```python
from build123d import *

# Parameters (mm, degrees)
Y_KSEKLIK_EKSTR_ZYON5_DEPTH = 4
Y_KSEKLIK_EKSTR_ZYON6_DEPTH = 40
RADYUS2_R                   = 1
KES_EKSTR_ZYON1_DEPTH       = 4
KES_EKSTR_ZYON2_DEPTH       = 35


with BuildPart() as part:
    # Çizim1 → Yükseklik-Ekstrüzyon5 (new body)
    with BuildSketch(Plane.XY):
        with BuildLine():
            Line((20, 0), (95, 0))
            ThreePointArc((95, 0), (100.857864376, -14.142135624), (115, -20))
            Line((115, -20), (115, -95))
            ThreePointArc((115, -95), (111.464466094, -96.464466094), (110, -100))
            Line((110, -100), (110, -170))
            Line((110, -170), (5, -170))
            Line((5, -170), (5, -100))
            ThreePointArc((5, -100), (3.535533906, -96.464466094), (0, -95))
            Line((0, -95), (0, -20))
            ThreePointArc((0, -20), (14.142135624, -14.142135624), (20, 0))
        make_face()
    extrude(amount=Y_KSEKLIK_EKSTR_ZYON5_DEPTH)

    # Çizim6 → Yükseklik-Ekstrüzyon6 (add)
    with BuildSketch(Plane.XY.offset(4)):
        Polygon((33.5, -4), (81.5, -4), (109.784271247, -32.284271247), (109.784271247, -87.284271247), (102.713203436, -94.355339059), (102.713203436, -154.355339059), (93.52081528, -163.547727215), (21.47918472, -163.547727215), (12.286796564, -154.355339059), (12.286796564, -94.355339059), (5.215728753, -87.284271247), (5.215728753, -32.284271247), align=None)
    extrude(amount=Y_KSEKLIK_EKSTR_ZYON6_DEPTH)

    # Radyus2
    radyus2_edges = [part.edges().sort_by_distance(p)[0] for p in [
        (20, 0, 2),
        (95, 0, 2),
        (115, -20, 2),
        (115, -95, 2),
        (110, -170, 2),
        (5, -170, 2),
        (0, -95, 2),
        (0, -20, 2),
        (95.642135624, -18.142135624, 4),
        (109.784271247, -32.284271247, 24),
        (57.5, -4, 4),
        (81.5, -4, 24),
        (19.357864376, -18.142135624, 4),
        (33.5, -4, 24),
        (5.215728753, -59.784271247, 4),
        (5.215728753, -32.284271247, 24),
        (8.751262658, -90.819805153, 4),
        (5.215728753, -87.284271247, 24),
        (12.286796564, -124.355339059, 4),
        (12.286796564, -94.355339059, 24),
        (16.882990642, -158.951533137, 4),
        (12.286796564, -154.355339059, 24),
        (57.5, -163.547727215, 4),
        (21.47918472, -163.547727215, 24),
        (98.117009358, -158.951533137, 4),
        (93.52081528, -163.547727215, 24),
        (102.713203436, -124.355339059, 4),
        (102.713203436, -154.355339059, 24),
        (106.248737342, -90.819805153, 4),
        (102.713203436, -94.355339059, 24),
        (109.784271247, -59.784271247, 4),
        (109.784271247, -87.284271247, 24),
        (95.642135624, -18.142135624, 44),
        (57.5, -4, 44),
        (19.357864376, -18.142135624, 44),
        (5.215728753, -59.784271247, 44),
        (8.751262658, -90.819805153, 44),
        (12.286796564, -124.355339059, 44),
        (16.882990642, -158.951533137, 44),
        (57.5, -163.547727215, 44),
        (98.117009358, -158.951533137, 44),
        (102.713203436, -124.355339059, 44),
        (106.248737342, -90.819805153, 44),
        (109.784271247, -59.784271247, 44),
    ]]
    fillet(radyus2_edges, radius=RADYUS2_R)

    # Çizim8 → Kes-Ekstrüzyon1 (cut)
    with BuildSketch(Plane(origin=(0, 0, 0), x_dir=(-1, 0, 0), z_dir=(0, 0, -1))):
        Polygon((-81.5, -5), (-33.5, -5), (-5.215728753, -33.284271247), (-5.215728753, -88.284271247), (-12.286796564, -95.355339059), (-12.286796564, -153.355339059), (-21.47918472, -162.547727215), (-93.52081528, -162.547727215), (-102.713203436, -153.355339059), (-102.713203436, -95.355339059), (-109.784271247, -88.284271247), (-109.784271247, -33.284271247), align=None)
    extrude(amount=-KES_EKSTR_ZYON1_DEPTH, mode=Mode.SUBTRACT)

    # Çizim9 → Kes-Ekstrüzyon2 (cut)
    with BuildSketch(Plane(origin=(0, 0, 4), x_dir=(-1, 0, 0), z_dir=(0, 0, -1))):
        Polygon((-80.5, -7), (-34.5, -7), (-6.922835534, -34.577164466), (-6.922835534, -86.577164466), (-14.701010127, -94.355339059), (-14.701010127, -150.355339059), (-22.47918472, -158.133513652), (-92.52081528, -158.133513652), (-100.298989873, -150.355339059), (-100.298989873, -94.355339059), (-108.077164466, -86.577164466), (-108.077164466, -34.577164466), align=None)
    extrude(amount=-KES_EKSTR_ZYON2_DEPTH, mode=Mode.SUBTRACT)


solid = part.part
```
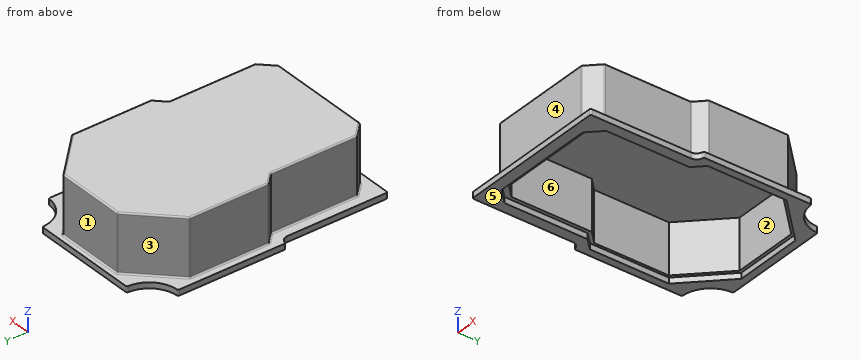
Verification items for the finished model (mm, model axes). Face numbers are marked on the shaded views. A direction names the side the tool comes from. Round coordinates to 2 decimals unless told otherwise and drop trailing zeros. Order: outer loops, then holes, each group sorted by start corner. A loop starts at its lowest first (then second) coordinate and runs counter-clockwise, first axis right, second up. Notation, with made-up numbers: (32, 52.5) - (72, 52.5) arc R23 cw to (72, 78.5) - close; hole circle Ø6 at (-26, 17.25). An arc over 180 degrees is marked (long way). Use CSV: the item, a comma, the result in double quotes. Start each with the question number.
1) Access from +Z, -Z, +X, -X, +Y, -Y to the whole of each face (thin tool, end or side, straight path). Record for the marked faces 1, 2 and 3.
2) Thickness scan on L1, parallel to X at y = -98.5, z = 10; L2, parallel to X at y = -44.5, z = 18.5; L3, parallel to Y at x = 41.5, z = 10. Record the ranges inside material, lowest first.
3) Go/stop test with flat-tipped pins: P1, Ø2, axis at x = 50.5, z = 2.5, coming from the +Y side; P2, Ø19, axis at x = 69, z = 24.5, coming from the +Y side; P3, Ø10, axis at x = 53, z = 27.5, coming from the -Y side; P4, Ø12, axis at y = -30, z = 32, coming from the -X side. Record where each tip stops, or that it passes through.
4) Section check A-A, the plane x = 73. Record the cut outline in (y, z), plus the area to 3 significant figures.
5) Mould release check, pull along Y, two halves, no side actions. Record for the marked faces 4, 5 and 6: +Y half, -Y half, draft (parallel to the pull), parting line (faces both ways), or undercut.
6) Section check B-B, the plane y = -58.5. Record the cut outline in (x, z), plus the area to 3 significant figures.
Answers:
1,face 1,"+Z, +X, -X, +Y"
1,face 2,"-Z"
1,face 3,"+Z, -X, +Y"
2,L1,"x = 12.29 to 14.7, 100.3 to 102.71"
2,L2,"x = 5.22 to 6.92, 108.08 to 109.78"
2,L3,"y = -163.55 to -158.13, -7 to -4"
3,P1,"stops at y = 0"
3,P2,"stops at y = -4"
3,P3,"stops at y = -163.55"
3,P4,"stops at x = 5.22"
4,outline,"(-170, 0) - (-162.55, 0) - (-162.55, 4) - (-158.13, 4) - (-158.13, 39) - (-7, 39) - (-7, 4) - (-5, 4) - (-5, 0) - (0, 0) - (0, 4) - (-3, 4) arc R1 cw to (-4, 5) - (-4, 43) arc R1 ccw to (-5, 44) - (-162.55, 44) arc R1 ccw to (-163.55, 43) - (-163.55, 5) arc R1 cw to (-164.55, 4) - (-170, 4) - close"
4,area,"1,140 mm²"
5,face 4,"-Y half"
5,face 5,"draft"
5,face 6,"undercut"
6,outline,"(0, 0) - (5.22, 0) - (5.22, 4) - (6.92, 4) - (6.92, 39) - (108.08, 39) - (108.08, 4) - (109.78, 4) - (109.78, 0) - (115, 0) - (115, 4) - (110.78, 4) arc R1 cw to (109.78, 5) - (109.78, 43) arc R1 ccw to (108.78, 44) - (6.22, 44) arc R1 ccw to (5.22, 43) - (5.22, 5) arc R1 cw to (4.22, 4) - (0, 4) - close"
6,area,"684 mm²"
